from build123d import *

# Parameters (mm, degrees)
F1_DEPTH       = 80
F2_R           = 9.4880271992
F3_DEPTH       = 600
F4_W           = 4.0547028184
F4_H           = 2.2076517344
F5_DEPTH       = 15
F6_R           = 8
F7_DEPTH       = 600
F9_START       = 50
F8_R           = 7.625
F9_DEPTH       = 570
F10_W          = 0.488139689
F10_H          = 8.393028751
F11_DEPTH      = 15
F13_DEPTH      = 25
F15_DEPTH      = 50
F17_DEPTH      = 295
F18_W          = 80
F18_H          = 61.0322915018
F19_DEPTH      = 10
F20_W          = 42.3060953617
F20_H          = 7.0626735687
F21_DEPTH      = 25
F22_W          = 33.6821526289
F22_H          = 16.1662399769
F23_DEPTH      = 25
F27_DEPTH      = 25
F28_R          = 5
F29_W          = 9.2532746494
F29_H          = 2.9556490481
F30_DEPTH      = 25
F30_DEPTH_BACK = 25
F31_R          = 1.8108941825
F32_DEPTH      = 25
F34_DEPTH      = 25
F35_W          = 14.8578360677
F35_H          = 28.517103754
F36_DEPTH      = 40


with BuildPart() as f1:
    # F0 (on Front) → F1 (new body)
    with BuildSketch(Plane.XZ):
        Polygon((0, 32.5182676315), (0, 0), (0, -28.3304974437), (43.5863435268, -28.3304974437), (43.5863435268, -20.3491598368), (7.9939365387, -20.3491598368), (7.9939365387, 0), (7.9939365387, 26.3243410736), (43.5863435268, 26.3243410736), (43.5863435268, 32.5182676315), align=None)
    extrude(amount=F1_DEPTH)

    # F2 (on face) → F3 (join)
    with BuildSketch(Plane.XY.offset(32.5182676315)):
        with Locations((32.2491303086, -37.8283821046)):
            Circle(F2_R)
    extrude(amount=F3_DEPTH)

    # F4 (on face) → F5 (cut)
    with BuildSketch(Plane.XY.offset(632.5182676315)):
        with Locations((22.9293145239, -37.5130698085)):
            Rectangle(F4_W, F4_H)
    extrude(amount=-F5_DEPTH, mode=Mode.SUBTRACT)

    # F6 (on face) → F7 (cut)
    with BuildSketch(Plane.XY.offset(632.5182676315)):
        with Locations((32.2491303086, -37.8283821046)):
            Circle(F6_R)
    extrude(amount=-F7_DEPTH, mode=Mode.SUBTRACT)


with BuildPart() as f9:
    # F8 (on face) → F9 (new body)
    with BuildSketch(Plane.XY.offset(32.5182676315).offset(F9_START)):
        with Locations((32.2491303086, -37.8283821046)):
            Circle(F8_R)
    extrude(amount=F9_DEPTH)

    # F10 (on face) → F11 (join)
    with BuildSketch(Plane.XY.offset(652.5182676315)):
        with Locations((31.1938934028, -27.710868977)):
            Rectangle(F10_W, F10_H)
    extrude(amount=-F11_DEPTH)

    # F12 (on face) → F13 (join)
    with BuildSketch(Plane.XY.offset(652.5182676315)):
        with BuildLine():
            ThreePointArc((24.8521837926, -35.977488472), (31.3166851855, -45.3961539757), (39.8741303086, -37.8283821046))
            ThreePointArc((39.8741303086, -37.8283821046), (39.8169021797, -36.8959369815), (39.6460768246, -35.977488472))
            Line((39.6460768246, -35.977488472), (24.8521837926, -35.977488472))
        make_face()
        with BuildLine():
            Line((24.8521837926, -35.977488472), (39.6460768246, -35.977488472))
            ThreePointArc((39.6460768246, -35.977488472), (32.2491303086, -30.2033821046), (24.8521837926, -35.977488472))
        make_face()
        with BuildLine():
            ThreePointArc((24.8521837926, -35.977488472), (32.2491303086, -30.2033821046), (39.6460768246, -35.977488472))
            Line((39.6460768246, -35.977488472), (39.6460768246, 264.022511528))
            Line((39.6460768246, 264.022511528), (24.8521837926, 264.022511528))
            Line((24.8521837926, 264.022511528), (24.8521837926, -35.977488472))
        make_face()
    extrude(amount=F13_DEPTH)

    # F14 (on face) → F15 (join)
    with BuildSketch(Plane.XY.offset(677.5182676315)):
        Polygon((154.8521837926, 264.022511528), (24.8521837926, 264.022511528), (-72.6417899132, 264.022511528), (-72.6417899132, -20.977488472), (154.8521837926, -20.977488472), align=None)
    extrude(amount=F15_DEPTH)

    # F16 (on face) → F17 (cut)
    with BuildSketch(Plane.XZ.offset(20.977488472)):
        Polygon((-52.7396649122, 686.2814426422), (154.8521837926, 727.5182676315), (-81.2070667744, 736.6052269936), (-72.6417899132, 692.2085285187), align=None)
    extrude(amount=-F17_DEPTH, mode=Mode.SUBTRACT)

    # F20 (on face) → F21 (join)
    with BuildSketch(Plane(origin=(0, 264.022511528, 0), x_dir=(-1, 0, 0), z_dir=(0, 1, 0))):
        with Locations((-93.7416106462, 696.6552138329)):
            Rectangle(F20_W, F20_H)
    extrude(amount=F21_DEPTH)

    # F22 (on face) → F23 (cut)
    with BuildSketch(Plane.XY.offset(700.1865506172)):
        with Locations((94.2212790251, 276.3699144125)):
            Rectangle(F22_W, F22_H)
    extrude(amount=-F23_DEPTH, mode=Mode.SUBTRACT)


with BuildPart() as f19:
    # F18 (on face) → F19 (new body)
    with BuildSketch(Plane.YZ.offset(43.5863435268)):
        with Locations((-40, 2.0021218807)):
            Rectangle(F18_W, F18_H)
    extrude(amount=F19_DEPTH)


with BuildPart() as f27:
    # F26 (on Top) → F27 (new body)
    with BuildSketch(Plane.XY):
        with BuildLine():
            Line((24.8369053006, 2), (17.3853386507, 2))
            ThreePointArc((17.3853386507, 2), (-17.5, 0), (17.3853386507, -2))
            Line((17.3853386507, -2), (24.8369053006, -2))
            Line((24.8369053006, -2), (25.3369053006, -2))
            Line((25.3369053006, -2), (25.3369053006, -1.5))
            Line((25.3369053006, -1.5), (25.3369053006, 1.5))
            Line((25.3369053006, 1.5), (25.3369053006, 2))
            Line((25.3369053006, 2), (24.8369053006, 2))
        make_face()
        with BuildLine():
            ThreePointArc((14.8817712447, -1.8795969301), (-15, 0), (14.8817712447, 1.8795969301))
            ThreePointArc((14.8817712447, 1.8795969301), (15.881113349, 1.6148969042), (16.9085127097, 1.5))
            Line((16.9085127097, 1.5), (17.4355957742, 1.5))
            Line((17.4355957742, 1.5), (24.8369053006, 1.5))
            Line((24.8369053006, 1.5), (24.8369053006, -1.5))
            Line((24.8369053006, -1.5), (17.4355957742, -1.5))
            Line((17.4355957742, -1.5), (16.9085127097, -1.5))
            ThreePointArc((16.9085127097, -1.5), (15.881113349, -1.6148969042), (14.8817712447, -1.8795969301))
        make_face(mode=Mode.SUBTRACT)
    extrude(amount=F27_DEPTH)

    # F28
    f28_edges = [f27.edges().sort_by_distance(p)[0] for p in [
        (17.385339, -2, 12.5),
        (17.385339, 2, 12.5),
    ]]
    fillet(f28_edges, radius=F28_R)

    # F29 (on Top) → F30 (cut, two sides)
    with BuildSketch(Plane.XY) as f30_sk:
        with Locations((24.9223280698, 0)):
            Rectangle(F29_W, F29_H)
    extrude(amount=-F30_DEPTH, mode=Mode.SUBTRACT)
    extrude(f30_sk.sketch, amount=F30_DEPTH_BACK, mode=Mode.SUBTRACT)

    # F31 (on face) → F32 (cut)
    with BuildSketch(Plane.XZ.offset(2)):
        with Locations((23.3601550405, 21.0856944323)):
            Circle(F31_R)
        with Locations((23.3601550405, 3.9143055677)):
            Circle(F31_R)
    extrude(amount=-F32_DEPTH, mode=Mode.SUBTRACT)

    # F33 (on Top) → F34 (join)
    with BuildSketch(Plane.XY):
        with BuildLine():
            Line((-33.1695042551, -16.8028511107), (-5.9619173408, -16.8028511107))
            ThreePointArc((-5.9619173408, -16.8028511107), (-6.6048434296, -16.5651949873), (-7.2380969958, -16.3028511107))
            Line((-7.2380969958, -16.3028511107), (-32.6695042551, -16.3028511107))
            Line((-32.6695042551, -16.3028511107), (-32.6695042551, 15.59525626))
            Line((-32.6695042551, 15.59525626), (-7.4055092994, 15.59525626))
            Line((-7.4055092994, 15.59525626), (-7.4055092994, 14.9921714968))
            ThreePointArc((-7.4055092994, 14.9921714968), (-7.2011649888, 15.0890530596), (-6.9955289917, 15.1831618859))
            Line((-6.9955289917, 15.1831618859), (-7.4055092994, 16.09525626))
            Line((-7.4055092994, 16.09525626), (-33.1695042551, 16.09525626))
            Line((-33.1695042551, 16.09525626), (-33.1695042551, 15.59525626))
            Line((-33.1695042551, 15.59525626), (-33.1695042551, -16.8028511107))
        make_face()
        with BuildLine():
            ThreePointArc((-7.2380969958, -16.3028511107), (-6.6048434296, -16.5651949873), (-5.9619173408, -16.8028511107))
            Line((-5.9619173408, -16.8028511107), (-5.633405689, -15.8583511929))
            ThreePointArc((-5.633405689, -15.8583511929), (-16.8329065642, -1.0255109398), (-7.4055092994, 14.9921714968))
            Line((-7.4055092994, 14.9921714968), (-7.4055092994, 15.59525626))
            Line((-7.4055092994, 15.59525626), (-32.6695042551, 15.59525626))
            Line((-32.6695042551, 15.59525626), (-32.6695042551, -16.3028511107))
            Line((-32.6695042551, -16.3028511107), (-7.2380969958, -16.3028511107))
        make_face()
    extrude(amount=F34_DEPTH)

    # F35 (on Top) → F36 (cut)
    with BuildSketch(Plane.XY):
        with Locations((-24.4145058095, 0.2095359378)):
            Rectangle(F35_W, F35_H)
    extrude(amount=F36_DEPTH, mode=Mode.SUBTRACT)


solid = f27.part
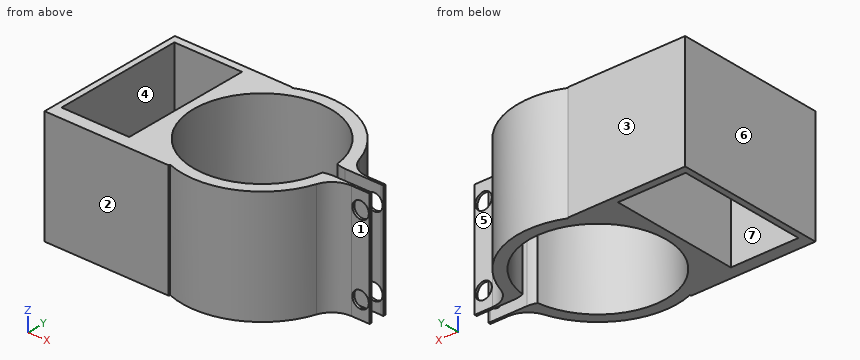
For this review, take the finished solid that the model builds, in its own axes (mm). Face numbers are marked on the shaded views. A direction names the side the tool comes from. Round coordinates to 2 decimals unless told otherwise and drop trailing zeros. Order: outer loops, then holes, each group sorted by start corner. A loop starts at its lowest first (then second) coordinate and runs counter-clockwise, first axis right, second up. Notation, with made-up numbers: M 59.25,88.5 L 118.25,88.5 A21 cw 118.25,112.5 Z; hole C -21,53.25 d4. An arc over 180 degrees is marked long. Use a Markdown table: item, result. Add a question column.
Item 1: Mouldability with a two-part tool opening along Y and no side actions: class the marked faces 5, 6 and 7 as released by +Y, released by -Y, zero draft, split by the parting line, or undercut.
Item 2: To check wall thickness, follow line 1 along Y through (x, z) = (-26, 14); line 2 along X through (y, z) = (11.5, 20.25); line 3 along X through (y, z) = (-12, 13.5). State the ranges of each line that lie inside material, in increasing order.
Item 3: Insertion check: pin 1 (3 mm diameter, centred on y = 9.5, z = 7.5, fed in from +X); pin 2 (2 mm diameter, centred on y = -9.5, z = 19, fed in from +X); pin 3 (10 mm diameter, centred on x = -11, z = 11, fed in from +Y); pin 4 (2 mm diameter, centred on x = 23.36, z = 3.91, fed in from -Y). Each pin has a flat end and moves straight along its axis. Give the tip position at first contact, or say it passes through.
Item 4: Add section D-D, the plane y = -7.5. Give the boundary of the cut face in (x, z).
Item 5: Add section B-B, the plane x = 0. Give the boundary of the cut face in (y, z).
Item 6: Tool access review of the marked faces 1, 2, 3 and 4: name each direction out of +Z, -Z, +X, -X, +Y, -Y from which nothing blocks a thin tool from reaching the whole face with its end or side.
Item 7: Add section A-A, the plane y = 0. Give the boundary of the cut face in (x, z).
Geometry results:
| question | item | result |
|---|---|---|
| 1 | face 5 | released by +Y |
| 1 | face 6 | zero draft |
| 1 | face 7 | undercut |
| 2 | line 1 | y = -16.8 to -14.05, 14.47 to 16.1 |
| 2 | line 2 | x = -33.17 to -31.84, -16.99 to -9.63, 9.63 to 13.19 |
| 2 | line 3 | x = -33.17 to -31.84, -16.99 to -9, 9 to 12.74 |
| 3 | pin 1 | stops at x = 15.56 |
| 3 | pin 2 | stops at x = 15.3 |
| 3 | pin 3 | stops at y = 16.44 |
| 3 | pin 4 | passes through |
| 4 | outline | M -33.17,0 L -31.84,0 L -31.84,25 L -33.17,25 Z; M -16.99,0 L -12.99,0 L -12.99,25 L -16.99,25 Z; M 12.99,0 L 15.81,0 L 15.81,25 L 12.99,25 Z |
| 5 | outline | M -17.5,0 L -15,0 L -15,25 L -17.5,25 Z; M 15,0 L 17.5,0 L 17.5,25 L 15,25 Z |
| 6 | face 1 | +Z, -Z, +X, -Y |
| 6 | face 2 | +Z, -Z, -X, -Y |
| 6 | face 3 | +Z, -Z, -X, +Y |
| 6 | face 4 | +Z, -Z |
| 7 | outline | M -33.17,0 L -31.84,0 L -31.84,25 L -33.17,25 Z; M -16.99,0 L -15,0 L -15,25 L -16.99,25 Z |
